Geometry: see drawing. Coordinates: mm, zero at the bounding-box minimum. A direction names the side the tool comes from. Give positions to 0.01 mm unless a question says otherwise; leave off trailing zeros. Write each loop counter-clockwise with the first axis right and the second up, starting at its lowest first coordinate (ties: lowest second). Pieces come first, ordered by that corner, then holes. Notation, with made-up numbers: M 64,-13 L 116,-13 A29 cw 116,17 Z; hole C 0,-13.5 d1. An arc over 180 degrees is marked long. Use a Markdown table: item, result. Add a question column.
1) Section C-C on x = 19.5. Return the cut outline in (y, z).
2) Section B-B on z = 9. Return the cut outline in (x, y), then the cut area to 3 significant figures.
3) Line query: line 1 (X direction, y = 3.5, z = 6); line 2 (Z direction, x = 10.5, y = 8); line 3 (Z direction, x = 6.5, y = 9.25). Output: solid intervals per line, ascending.
4) Set-up query: the marked faces 1, 2 and 3. Return all of +Z, -Z, +X, -X, +Y, -Y with unobstructed straight access to the full face (end or side cutting, diameter ignored); none if empty.
5) Pin query (flat end, axial travel): pin 1 (5 mm diameter, centred on x = 10, z = 15, fed in from -Y); pin 2 (8 mm diameter, centred on y = 14.5, z = 16, fed in from -X); pin 3 (3 mm diameter, centred on x = 6.5, z = 5.5, fed in from +Y) (1 decimal); pin 4 (1 mm diameter, centred on x = 3, z = 10.5, fed in from +Y). Return the tip coordinate at first contact, or that it passes through.
6) Section A-A on y = 8. Return the cut outline in (x, z).
7) Section D-D on x = 3.25. Return the cut outline in (y, z).
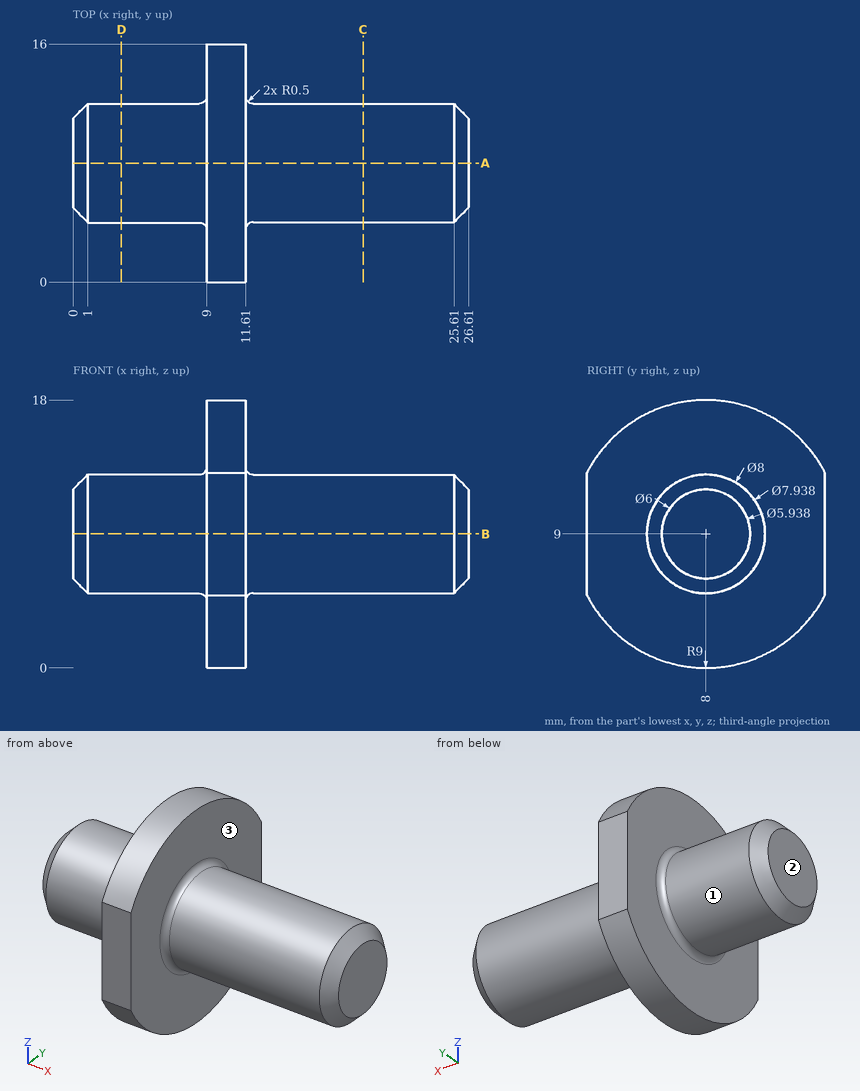
Found:
| question | item | result |
|---|---|---|
| 1 | outline | C 8,9 d7.94 |
| 2 | outline | M 0,5 L 1,4 L 8.5,4 A0.5 cw 9,3.5 L 9,0 L 11.61,0 L 11.61,3.53 A0.5 cw 12.11,4.03 L 25.61,4.03 L 26.61,5.03 L 26.61,10.97 L 25.61,11.97 L 12.11,11.97 A0.5 cw 11.61,12.47 L 11.61,16 L 9,16 L 9,12.5 A0.5 cw 8.5,12 L 1,12 L 0,11 Z |
| 2 | area | 231 mm² |
| 3 | line 1 | 9 to 11.61 |
| 3 | line 2 | 0 to 18 |
| 3 | line 3 | 5.2 to 12.8 |
| 4 | face 1 | -X |
| 4 | face 2 | +Z, -Z, -X, +Y, -Y |
| 4 | face 3 | +X |
| 5 | pin 1 | y = 0 |
| 5 | pin 2 | x = 9 |
| 5 | pin 3 | y = 11.5 |
| 5 | pin 4 | y = 11.87 |
| 6 | outline | M 0,6 L 1,5 L 8.5,5 A0.5 cw 9,4.5 L 9,0 L 11.61,0 L 11.61,4.53 A0.5 cw 12.11,5.03 L 25.61,5.03 L 26.61,6.03 L 26.61,11.97 L 25.61,12.97 L 12.11,12.97 A0.5 cw 11.61,13.47 L 11.61,18 L 9,18 L 9,13.5 A0.5 cw 8.5,13 L 1,13 L 0,12 Z |
| 7 | outline | C 8,9 d8 |
